```python
from build123d import *

# Parameters (mm, degrees)
SKETCH1_W           = 26
SKETCH1_H           = 46
BOSS_EXTRUDE1_DEPTH = 5.8
CUT_EXTRUDE1_START  = -0.4
SKETCH2_W           = 24.7
SKETCH2_H           = 45
CUT_EXTRUDE1_DEPTH  = 5
SKETCH3_W           = 30.3
SKETCH3_H           = 54.5
BOSS_EXTRUDE2_DEPTH = 1
SKETCH4_W           = 1
SKETCH4_H           = 54.5
BOSS_EXTRUDE3_DEPTH = 8
SKETCH5_W           = 29.3
SKETCH5_H           = 1
BOSS_EXTRUDE4_DEPTH = 8
SKETCH6_W           = 1
SKETCH6_H           = 53.5
BOSS_EXTRUDE5_DEPTH = 8
SKETCH7_W           = 28.3
SKETCH7_H           = 1
BOSS_EXTRUDE6_DEPTH = 8
SKETCH8_W           = 19.840922592
SKETCH8_H           = 47.393191015
CUT_EXTRUDE2_DEPTH  = 2
SKETCH9_W           = 24.7
SKETCH9_H           = 25.217114116
CUT_EXTRUDE3_DEPTH  = 1


with BuildPart() as part:
    # Sketch1 → Boss-Extrude1 (new body)
    with BuildSketch(Plane(origin=(0, 0, 0), x_dir=(1, 0, 0), z_dir=(0, 1, 0))):
        with Locations((13, 23)):
            Rectangle(SKETCH1_W, SKETCH1_H)
    extrude(amount=BOSS_EXTRUDE1_DEPTH)

    # Sketch2 → Cut-Extrude1 (cut)
    with BuildSketch(Plane(origin=(0, 5.8, 0), x_dir=(1, 0, 0), z_dir=(0, 1, 0)).offset(CUT_EXTRUDE1_START)):
        with Locations((13, 22)):
            Rectangle(SKETCH2_W, SKETCH2_H)
    extrude(amount=-CUT_EXTRUDE1_DEPTH, mode=Mode.SUBTRACT)

    # Sketch3 → Boss-Extrude2 (add)
    with BuildSketch(Plane(origin=(0, 5.8, 0), x_dir=(1, 0, 0), z_dir=(0, 1, 0))):
        with Locations((12.858896044, 21.143191015)):
            Rectangle(SKETCH3_W, SKETCH3_H)
    extrude(amount=BOSS_EXTRUDE2_DEPTH)

    # Sketch4 → Boss-Extrude3 (add)
    with BuildSketch(Plane.XZ.offset(-5.8)):
        with Locations((-1.791103956, -21.143191015)):
            Rectangle(SKETCH4_W, SKETCH4_H)
    extrude(amount=BOSS_EXTRUDE3_DEPTH)

    # Sketch5 → Boss-Extrude4 (add)
    with BuildSketch(Plane.XZ.offset(-5.8)):
        with Locations((13.358896044, 5.606808985)):
            Rectangle(SKETCH5_W, SKETCH5_H)
    extrude(amount=BOSS_EXTRUDE4_DEPTH)

    # Sketch6 → Boss-Extrude5 (add)
    with BuildSketch(Plane.XZ.offset(-5.8)):
        with Locations((27.508896044, -21.643191015)):
            Rectangle(SKETCH6_W, SKETCH6_H)
    extrude(amount=BOSS_EXTRUDE5_DEPTH)

    # Sketch7 → Boss-Extrude6 (add)
    with BuildSketch(Plane.XZ.offset(-5.8)):
        with Locations((12.858896044, -47.893191015)):
            Rectangle(SKETCH7_W, SKETCH7_H)
    extrude(amount=BOSS_EXTRUDE6_DEPTH)

    # Sketch8 → Cut-Extrude2 (cut)
    with BuildSketch(Plane.XZ):
        with Locations((12.675861703, -23.696595508)):
            Rectangle(SKETCH8_W, SKETCH8_H)
    extrude(amount=-CUT_EXTRUDE2_DEPTH, mode=Mode.SUBTRACT)

    # Sketch9 → Cut-Extrude3 (cut)
    with BuildSketch(Plane.XZ):
        with Locations((13.034968762, -12.580450922)):
            Rectangle(SKETCH9_W, SKETCH9_H)
    extrude(amount=-CUT_EXTRUDE3_DEPTH, mode=Mode.SUBTRACT)


solid = part.part
```
CAD build for the part. Positions are in the model's coordinates, mm. A direction names the side the tool comes from. Round coordinates to 2 decimals unless told otherwise and drop trailing zeros. Order: outer loops, then holes, each group sorted by start corner. A loop starts at its lowest first (then second) coordinate and runs counter-clockwise, first axis right, second up.
Item 1: Saw through at D-D on x = 1.5. Write the cut outline in (y, z).
Item 2: Saw through at B-B on x = 12. Write the cut outline in (y, z), then the cut area to 3 significant figures.
Item 3: Mould opens along X. For faces 4 (the face through (25.35, 3, -22)), 5 (the face through (13, 6.8, -22)), 6 (the face through (-2.291, 2, -22)) say: pulls with the +X half, pulls with the -X half, needs draft (parallel to the pull), parting line crosses it, or undercut.
Item 4: Probe line 1 along Z through (x, y) = (12, 3.25); line 2 along X through (y, z) = (0.5, -31); line 3 along Z through (x, y) = (7, 5.75). List the from-to ranges inside material, lowest first.
Item 5: Saw through at A-A on y = 3.75. Write the cut outline in (x, z).
Item 6: Tool access for faces 1 (the face through (27.4, -2.2, -12.9)), 2 (the face through (25.385, 0.5, -12.8)), 3 (the face through (24, 0.4, -35)): list every direction of +Z, -Z, +X, -X, +Y, -Y with a clear straight run to the whole face (end or side of a thin tool).
Item 7: Pin check, flat tips, straight feed: pin 1 (1 mm diameter, centred on x = 24, z = -24, fed in from -Y); pin 2 (2.5 mm diameter, centred on x = 24.5, z = -27, fed in from -Y); pin 3 (1.6 mm diameter, centred on x = 10.5, z = -45.5, fed in from -Y). Stop position of each tip, or through.
Reported:
1. outline: (-2.2, -48.39) - (6.8, -48.39) - (6.8, 6.11) - (-2.2, 6.11) - (-2.2, 5.11) - (5.8, 5.11) - (5.8, 0) - (5.4, 0) - (5.4, -44.5) - (0.4, -44.5) - (0.4, -25.19) - (0, -25.19) - (0, -46) - (5.8, -46) - (5.8, -47.39) - (-2.2, -47.39) - close
2. outline: (-2.2, -48.39) - (6.8, -48.39) - (6.8, 6.11) - (-2.2, 6.11) - (-2.2, 5.11) - (5.8, 5.11) - (5.8, 0) - (5.4, 0) - (5.4, -44.5) - (2, -44.5) - (2, -46) - (5.8, -46) - (5.8, -47.39) - (-2.2, -47.39) - close
2. area: 94.0 mm2
3. face 4: undercut
3. face 5: needs draft
3. face 6: pulls with the -X half
4. line 1: z = -48.39 to -47.39, -46 to -44.5, 5.11 to 6.11
4. line 2: x = -2.29 to -1.29, 0 to 0.65, 25.35 to 26, 27.01 to 28.01
4. line 3: z = -48.39 to -47.39, -46 to 0, 5.11 to 6.11
5. outline: (-2.29, -48.39) - (28.01, -48.39) - (28.01, 6.11) - (-2.29, 6.11) - close; (0, -46) - (26, -46) - (26, 0) - (25.35, 0) - (25.35, -44.5) - (0.65, -44.5) - (0.65, 0) - (0, 0) - close; hole (-1.29, -47.39) - (27.01, -47.39) - (27.01, 5.11) - (-1.29, 5.11) - close
6. face 1: +Z, -Z, +X, -X, -Y
6. face 2: -Y
6. face 3: none
7. pin 1: stops at y = 5.4
7. pin 2: stops at y = 0
7. pin 3: stops at y = 2
